Drawing for the job (mm, zero at the part's lowest x, y, z). Give positions to 0.01 mm unless a question says otherwise; leave off trailing zeros. Order: outer loops, then holes, each group sorted by start corner. A loop starts at its lowest first (then second) coordinate and runs counter-clockwise, first axis right, second up. Notation, with made-up numbers: (-18, 7) - (-8, 7) arc R16 ccw to (-8, 37) - close; hole circle Ø7 at (40, 87.25). An arc over 180 degrees is marked (long way). Use a Markdown table: item, result.
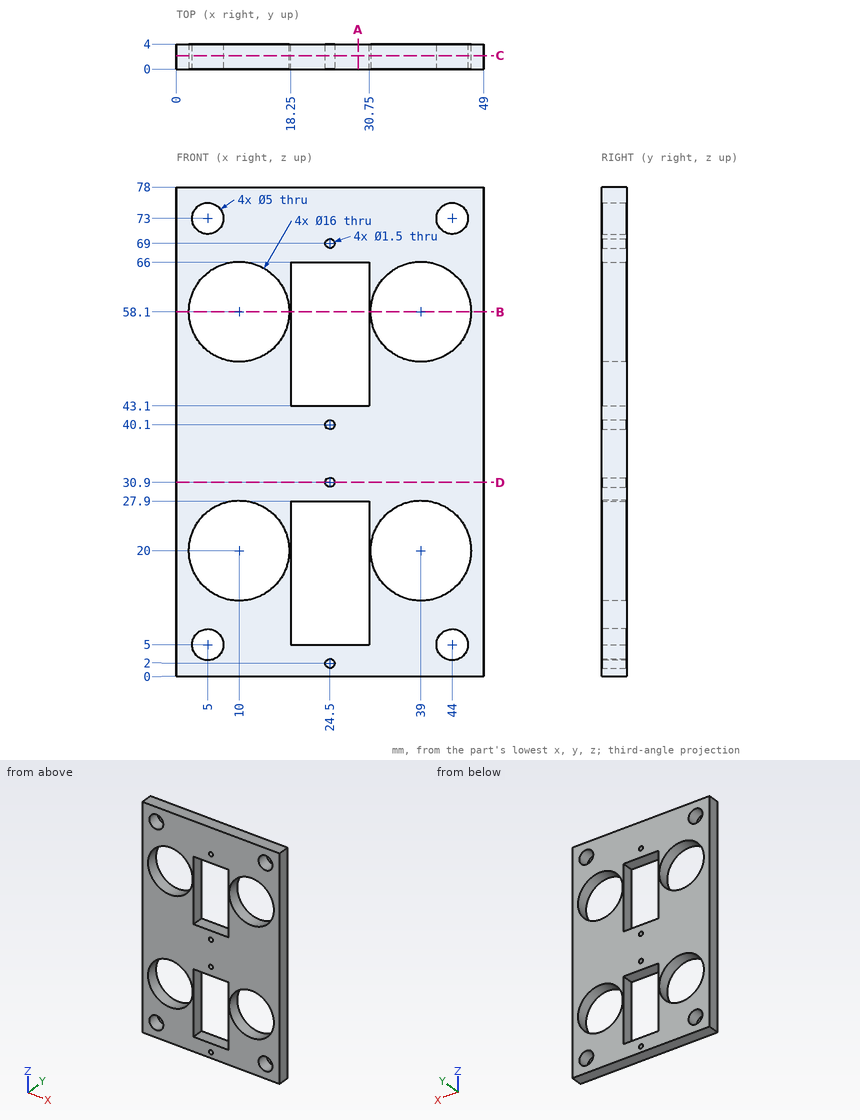
1) Slice it at D-D (z = 30.9). Write the cut outline in (x, y), and give its area (3 significant figures).
Computed:
| item | result |
|---|---|
| outline | (0, 0) - (23.75, 0) - (23.75, 4) - (0, 4) - close; (25.25, 0) - (49, 0) - (49, 4) - (25.25, 4) - close |
| area | 190 mm² |
2) Slice it at C-C (y = 2.15). State how many separate pieces and enclosed holes the cut face has, and give its area (3 significant figures).
Computed:
| item | result |
|---|---|
| separate pieces | 1 |
| enclosed holes | 14 |
| area | 2,360 mm² |
3) Wall check: line 1 (Z direction, x = 39, y = 2); line 2 (Z direction, x = 29.5, y = 1.5); line 3 (X direction, y = 1, z = 24). Give the ranges that are in metal, low to high. Write a range as from..to.
Computed:
| item | result |
|---|---|
| line 1 | z = 0..12, 28..50.1, 66.1..78 |
| line 2 | z = 0..5, 27.9..43.1, 66..78 |
| line 3 | x = 0..3.07, 16.93..18.25, 30.75..32.07, 45.93..49 |
4) Slice it at B-B (z = 58.1). Write the cut outline in (x, y).
Computed:
| item | result |
|---|---|
| outline | (0, 0) - (2, 0) - (2, 4) - (0, 4) - close; (18, 0) - (18.25, 0) - (18.25, 4) - (18, 4) - close; (30.75, 0) - (31, 0) - (31, 4) - (30.75, 4) - close; (47, 0) - (49, 0) - (49, 4) - (47, 4) - close |
5) Slice it at A-A (x = 29). Write the cut outline in (y, z).
Computed:
| item | result |
|---|---|
| outline | (0, 0) - (4, 0) - (4, 5) - (0, 5) - close; (0, 27.9) - (4, 27.9) - (4, 43.1) - (0, 43.1) - close; (0, 66) - (4, 66) - (4, 78) - (0, 78) - close |
